Can you work these out from the model? Positions are in its coordinate system, mm. Face numbers are marked on the shaded views. A direction names the side the tool comes from. Give positions to 0.01 mm unless a question says otherwise; leave off trailing zeros. Order: outer loops, then holes, each group sorted by start corner. A loop starts at its lowest first (then second) coordinate and runs counter-clockwise, first axis right, second up. Notation, with made-up numbers: M 42.5,47.5 L 95.5,47.5 A30 cw 95.5,71.5 Z; hole C 10.25,73 d1. An arc over 180 degrees is marked long. Answer as a JSON object with one key per item and string values.
```python
from build123d import *

# Parameters (mm, degrees)
F0_R     = 2.6924
F1_DEPTH = 1.905
F2_R     = 0.889
F3_R     = 1.397
F4_DEPTH = 8.89
F5_SIZE  = 1.27


with BuildPart() as f1:
    # F0 (on Top) → F1 (new body)
    with BuildSketch(Plane.XY):
        Circle(F0_R)
    extrude(amount=F1_DEPTH)

    # F2
    f2_edges = [f1.edges().sort_by_distance(p)[0] for p in [
        (-2.6924, 0, 1.905),
    ]]
    fillet(f2_edges, radius=F2_R)

    # F3 (on Top) → F4 (join)
    with BuildSketch(Plane.XY):
        Circle(F3_R)
    extrude(amount=-F4_DEPTH)

    # F5
    f5_edges = [f1.edges().sort_by_distance(p)[0] for p in [
        (-1.397, 0, -8.89),
    ]]
    chamfer(f5_edges, length=F5_SIZE)


solid = f1.part
```
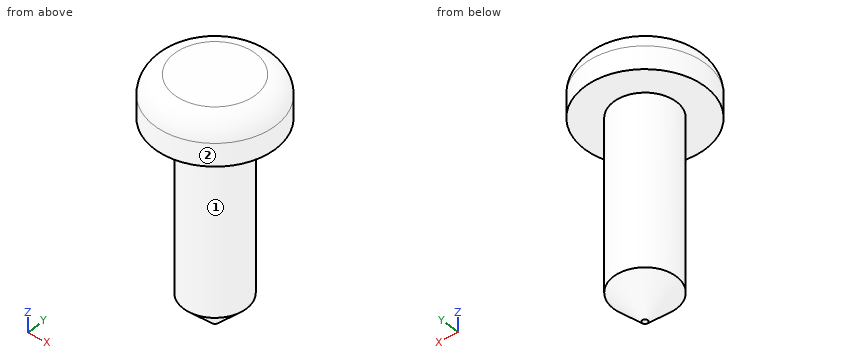
1) I need wall thicknesses on L1, parallel to Z at x = -1.35, y = 0.85 (3 decimals); L2, parallel to Z at x = -0.3, y = 2.2; L3, parallel to X at y = 0.8, z = -2.5. Which ranges of each line are inside material? Lowest first, please.
Results found:
{"L1": "z = 0 to 1.905", "L2": "z = 0 to 1.8", "L3": "x = -1.15 to 1.15"}
2) For the marked faces 1 and 2, which set-ups out of +Z, -Z, +X, -X, +Y, -Y let a thin tool reach every point of the face, with its end or its side?
Results found:
{"face 1": "-Z", "face 2": "+Z, -Z"}
3) I'm going to push flat-ended pins straight in: pin 1 Ø1 at (x, y) = (1.5, 1) entering from -Z; pin 2 Ø2 at (x, y) = (1.5, -1) entering from -Z. Where does each tip first touch, or does it pass through?
Results found:
{"pin 1": "stops at z = -7.71", "pin 2": "stops at z = -8.21"}
4) I want a section at C-C on z = -1.5. Write out the boundary of the cut face in (x, y), and give its area (3 significant figures).
Results found:
{"outline": "C 0,0 d2.79", "area": "6.13 mm²"}
5) I want a section at A-A on y = 0. Write out the boundary of the cut face in (x, z) (3 decimals).
Results found:
{"outline": "M -2.692,0 L -1.397,0 L -1.397,-7.62 L -0.127,-8.89 L 0.127,-8.89 L 1.397,-7.62 L 1.397,0 L 2.692,0 L 2.692,1.016 A0.889 ccw 1.803,1.905 L -1.803,1.905 A0.889 ccw -2.692,1.016 Z"}
